Part model, mm, in its own coordinate system. A direction names the side the tool comes from. Round coordinates to 2 decimals unless told otherwise and drop trailing zeros. Write each loop counter-clockwise with the first axis right and the second up, starting at its lowest first coordinate (ties: lowest second). Pieces come first, ordered by that corner, then holes. Notation, with made-up numbers: M 31.25,51 L 84.25,51 A22 cw 84.25,60 Z; hole C 12,76.25 d4. An arc over 180 degrees is marked long. Use a Markdown table: item, result. Add a question column.
1) Slice it at C-C on y = 7. Write the cut outline in (x, z).
2) Drop flat-ended pins along their axis: P1, Ø5, axis at y = 7, z = -5, coming from the -X side; P2, Ø5, axis at x = 4, z = -5, coming from the -Y side; P3, Ø4, axis at x = 10, y = 21.5, coming from the +Z side. Give the stop position or say it passes through.
3) Which spindle directions (+Z, -Z, +X, -X, +Y, -Y) get a long thin tool onto all of the face, cutting with end or side? Do faces 1 (the face through (3, 4, 0)), 2 (the face through (0, 0, 0)). Say none if no direction does.
4) Slice it at A-A on x = 0. Write the cut outline in (y, z).
5) Slice it at B-B on z = 0. Write the cut outline in (x, y).
6) Wall check: probe 1 along Y at (x, z) = (-4.75, 6); probe 2 along Z at (x, y) = (0, 9.5); probe 3 along X at (y, z) = (19.5, -4.5). Give the ranges that are in metal, low to high.
7) Slice it at D-D on y = 17. Write the cut outline in (x, z).
Autodesk Inventor part; units mm, degrees
ref_plane "YZ Plane" through (0, 0, 0) normal (1, 0, 0) x (0, 1, 0)
ref_plane "XZ Plane" through (0, 0, 0) normal (0, 1, 0) x (-1, 0, 0)
ref_plane "XY Plane" through (0, 0, 0) normal (0, 0, 1) x (1, 0, 0)
sketch "Sketch1" plane through (0, 0, 0) normal (0, 1, 0) x (-1, 0, 0)
  circle A0 centre (0, 0) radius 3
  dimension "d2" = 6
extrude "Extrusion1" add sketch "Sketch1" along normal blind 43.1
thread "Thread1"
sketch "Sketch3" plane through (0, 43.1, 0) normal (0, 1, 0) x (1, 0, 0)
  circle A0 centre (0, 0) radius 14.5
  dimension "d7" = 29
extrude "Extrusion2" add sketch "Sketch3" against normal blind 28.6
sketch "Sketch4" plane through (0, 43.1, 0) normal (0, 1, 0) x (1, 0, 0)
  circle A0 centre (0, 0) radius 3.95
  dimension "d10" = 7.9
extrude "Extrusion3" add sketch "Sketch4" against normal blind 35.6
fillet "Fillet1" radius 2 2 edges at (-14.5, 14.5, 0) (-14.5, 43.1, 0)
properties part number "bldc MOTOR"
Entries:
| question | item | result |
|---|---|---|
| 1 | outline | C 0,0 d6 |
| 2 | P1 | stops at x = -3.02 |
| 2 | P2 | stops at y = 7.5 |
| 2 | P3 | stops at z = 12.09 |
| 3 | face 1 | -Y |
| 3 | face 2 | +Z, -Z, +X, -X, -Y |
| 4 | outline | M 0,-3 L 7.5,-3 L 7.5,-3.95 L 14.5,-3.95 L 14.5,-12.5 A2 ccw 16.5,-14.5 L 41.1,-14.5 A2 ccw 43.1,-12.5 L 43.1,12.5 A2 ccw 41.1,14.5 L 16.5,14.5 A2 ccw 14.5,12.5 L 14.5,3.95 L 7.5,3.95 L 7.5,3 L 0,3 Z |
| 5 | outline | M -14.5,16.5 A2 ccw -12.5,14.5 L -3.95,14.5 L -3.95,7.5 L -3,7.5 L -3,0 L 3,0 L 3,7.5 L 3.95,7.5 L 3.95,14.5 L 12.5,14.5 A2 ccw 14.5,16.5 L 14.5,41.1 A2 ccw 12.5,43.1 L -12.5,43.1 A2 ccw -14.5,41.1 Z |
| 6 | probe 1 | y = 14.5 to 43.1 |
| 6 | probe 2 | z = -3.95 to 3.95 |
| 6 | probe 3 | x = -13.78 to 13.78 |
| 7 | outline | C 0,0 d29 |
